Input: part model. Units: mm. Frame: model coordinates. Face numbers are marked on the shaded views. A direction names the side the tool comes from. Coordinates: 2 decimals unless noted, no trailing zeros. Write each loop counter-clockwise with the first axis right and the second up, starting at its lowest first coordinate (ties: lowest second). Pieces come first, ordered by that corner, then holes. Notation, with made-up numbers: M -10,-40 L 29,-40 A21 ccw 29,-21 Z; hole C -5,31.5 d11. An arc over 180 degrees is marked long. Use CSV: the item, a comma, the result in double quotes.
```python
from build123d import *

# Parameters (mm, degrees)
SKETCH5_W            = 25
SKETCH5_H            = 20
BOSS_EXTRUDE3_DEPTH  = 2
SKETCH6_W            = 25
SKETCH6_H            = 2
BOSS_EXTRUDE4_DEPTH  = 16
BOSS_EXTRUDE5_DEPTH  = 2
BOSS_EXTRUDE6_DEPTH  = 1
SKETCH9_R            = 1.63
CUT_EXTRUDE2_DEPTH   = 23.632940596
FILLET1_R            = 1
SKETCH10_R           = 307
SKETCH10_R_2         = 297
CUT_EXTRUDE3_DEPTH   = 33.388269481
FILLET1_OF_MIRROR3_R = 1


with BuildPart() as part:
    # Sketch5 → Boss-Extrude3 (new body)
    with BuildSketch(Plane(origin=(0, 0, 0), x_dir=(1, 0, 0), z_dir=(0, 1, 0))):
        Rectangle(SKETCH5_W, SKETCH5_H)
    boss_extrude3 = extrude(amount=BOSS_EXTRUDE3_DEPTH)

    # Sketch6 → Boss-Extrude4 (add)
    with BuildSketch(Plane(origin=(0, 2, 0), x_dir=(1, 0, 0), z_dir=(0, 1, 0))):
        with Locations((0, 9)):
            Rectangle(SKETCH6_W, SKETCH6_H)
    boss_extrude4 = extrude(amount=BOSS_EXTRUDE4_DEPTH)

    # Sketch7 → Boss-Extrude5 (add)
    with BuildSketch(Plane(origin=(12.5, 0, 0), x_dir=(0, 0, -1), z_dir=(1, 0, 0))):
        Polygon((8, 18), (-10, 2), (8, 2), align=None)
    boss_extrude5 = extrude(amount=-BOSS_EXTRUDE5_DEPTH)

    # Sketch8 → Boss-Extrude6 (add)
    with BuildSketch(Plane.ZY.offset(12.5)):
        Polygon((-8, 18), (-8, 2), (10, 2), align=None)
    boss_extrude6 = extrude(amount=-BOSS_EXTRUDE6_DEPTH)

    # Sketch9 → Cut-Extrude2 (cut, symmetric)
    with BuildSketch(Plane(origin=(0, 2, 0), x_dir=(1, 0, 0), z_dir=(0, 1, 0))):
        with Locations(Location((-0.5, 3, 0), (0, 0, 270))):
            Circle(SKETCH9_R)
    cut_extrude2 = extrude(amount=CUT_EXTRUDE2_DEPTH, both=True, mode=Mode.SUBTRACT)

    # Fillet1
    fillet1_edges = [part.edges().sort_by_distance(p)[0] for p in [
        (10.5, 2, 1),
        (-0.5, 2, -8),
        (-11.5, 2, 1),
    ]]
    fillet(fillet1_edges, radius=FILLET1_R)

    # Sketch10 → Cut-Extrude3 (cut, through all)
    with BuildSketch(Plane(origin=(12.5, 0, 0), x_dir=(0, 0, -1), z_dir=(1, 0, 0))):
        with Locations((-287, 0)):
            Circle(SKETCH10_R)
        with Locations((-287, 0)):
            Circle(SKETCH10_R_2, mode=Mode.SUBTRACT)
    cut_extrude3 = extrude(amount=-CUT_EXTRUDE3_DEPTH, mode=Mode.SUBTRACT)


with BuildPart() as mirror3_1:
    # Mirror3: Boss-Extrude3, Boss-Extrude4, Boss-Extrude5, Boss-Extrude6 across plane
    add(boss_extrude3.mirror(Plane(origin=(-12.5, 2, -10), x_dir=(0, 0, 1), z_dir=(1, 0, 0))))
    add(boss_extrude4.mirror(Plane(origin=(-12.5, 2, -10), x_dir=(0, 0, 1), z_dir=(1, 0, 0))))
    add(boss_extrude5.mirror(Plane(origin=(-12.5, 2, -10), x_dir=(0, 0, 1), z_dir=(1, 0, 0))))
    add(boss_extrude6.mirror(Plane(origin=(-12.5, 2, -10), x_dir=(0, 0, 1), z_dir=(1, 0, 0))))

    # Mirror3 2: Cut-Extrude2, Cut-Extrude3 across plane
    add(cut_extrude2.mirror(Plane(origin=(-12.5, 2, -10), x_dir=(0, 0, 1), z_dir=(1, 0, 0))), mode=Mode.SUBTRACT)
    add(cut_extrude3.mirror(Plane(origin=(-12.5, 2, -10), x_dir=(0, 0, 1), z_dir=(1, 0, 0))), mode=Mode.SUBTRACT)

    # Fillet1 of Mirror3
    fillet1_of_mirror3_edges = [mirror3_1.edges().sort_by_distance(p)[0] for p in [
        (-35.5, 2, 1),
        (-24.5, 2, -8),
        (-13.5, 2, 1),
    ]]
    fillet(fillet1_of_mirror3_edges, radius=FILLET1_OF_MIRROR3_R)


with BuildPart() as part_1:
    add(part.part)

    # Mirror3 united with what the copies touc: union Mirror3_1
    add(mirror3_1.part)


solid = part_1.part
```
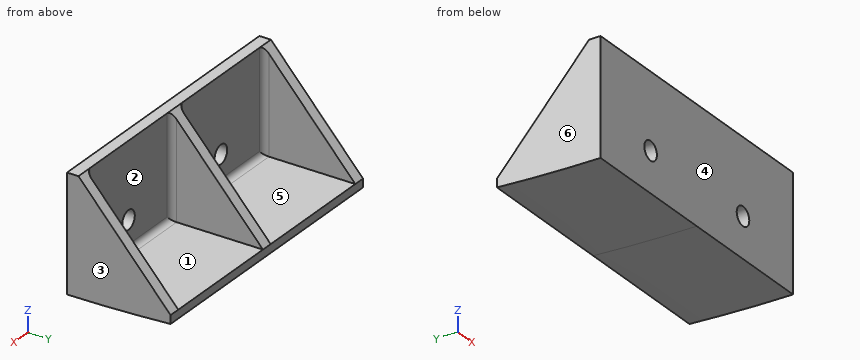
1. Contact query for flat-ended pins moving along their axis: pin 1 Ø3.5 at (x, z) = (-0.5, -3) entering from +Y; pin 2 Ø4.5 at (x, y) = (5, 10.5) entering from +Z; pin 3 Ø3 at (x, y) = (-7.5, 4.5) entering from -Z. Output: stop coordinate, or through.
Resolved:
pin 1,"stops at y = 2"
pin 2,"stops at z = -8"
pin 3,"stops at z = -9.98"
2. Section A-A (x = -24.5). Return loops of the section in (y, z), then the cut area to 3 significant figures.
Resolved:
outline,"M 0,-10 A297 ccw 18,-9.45 L 18,-8 L 3,-8 A1 cw 2,-7 L 2,-4.63 L 0,-4.63 Z; M 0,-1.37 L 2,-1.37 L 2,10 L 0,10 Z"
area,"62.4 mm^2"
3. Section C-C (y = 5.25). Return loops of the section in (x, z).
Resolved:
outline,"M -37.5,-9.95 L 12.5,-9.95 L 12.5,6.34 L 10.5,6.34 L 10.5,-8 L -11.5,-8 L -11.5,6.34 L -13.5,6.34 L -13.5,-8 L -35.5,-8 L -35.5,6.34 L -37.5,6.34 Z"
4. Access query for the marked faces 5 and 6. Directions: +Z, -Z, +X, -X, +Y, -Y. A direction counts if a zero-diameter tool reaches every point of the face in a straight line with its end or side. Return the directions, or none.
Resolved:
face 5,"+Z, +Y"
face 6,"+Z, -Z, -X, +Y, -Y"
5. Section B-B (x = 7). Return loops of the section in (y, z), then the cut area to 3 significant figures.
Resolved:
outline,"M 0,-10 A297 ccw 18,-9.45 L 18,-8 L 3,-8 A1 cw 2,-7 L 2,10 L 0,10 Z"
area,"68.9 mm^2"
6. Mould query, pull axis X, two halves, no side actions, for the marked faces 1, 2, 3 and 4. Classes: pulls with the +X half, pulls with the -X half, needs draft (parallel to the pull), parting line crosses it, or undercut.
Resolved:
face 1,"undercut"
face 2,"undercut"
face 3,"pulls with the +X half"
face 4,"needs draft"
7. Section D-D (z = -3). Return loops of the section in (x, y).
Resolved:
outline,"M -37.5,0 L -26.13,0 L -26.13,2 L -34.5,2 A1 cw -35.5,3 L -35.5,13.56 L -37.5,13.56 Z; M -22.87,0 L -2.13,0 L -2.13,2 L -10.5,2 A1 cw -11.5,3 L -11.5,13.56 L -13.5,13.56 L -13.5,3 A1 cw -14.5,2 L -22.87,2 Z; M 1.13,0 L 12.5,0 L 12.5,13.56 L 10.5,13.56 L 10.5,3 A1 cw 9.5,2 L 1.13,2 Z"
8. Material intervals for line 1 (X direction, y = 0.5, z = -3); line 2 (X direction, y = 6, z = 2); line 3 (Y direction, x = -34.5, z = 7.5), sorted ascending. Write a range as [from, to].
Resolved:
line 1,"x = [-37.5, -26.13], [-22.87, -2.13], [1.13, 12.5]"
line 2,"x = [-37.5, -35.5], [-13.5, -11.5], [10.5, 12.5]"
line 3,"y = [0, 2]"
